Part model, mm, in its own coordinate system. A direction names the side the tool comes from. Coordinates: 2 decimals unless noted, no trailing zeros. Loops run counter-clockwise (first coordinate to the right, second up) from the corner with the lowest first, then second, coordinate; pieces in that order, holes last. Notation, with made-up numbers: (22, 22.25) -> (46, 22.25) arc R20 ccw to (46, 59.25) -> close; hole circle Ø4 at (-31, 39). An arc over 180 degrees is marked (long way). One line per question, with ' | ' between items. Start each with the question number.
1) Cut at B-B (z = -3.75). List the corners of the cut face in (x, y), plus the area to 3 significant figures.
2) Cut at D-D (y = 1.45). Count the separate pieces of the cut face and the enclosed holes in it, plus the area to 3 significant figures.
3) Cut at C-C (z = -49). List the corners of the cut face in (x, y).
4) Two-plate mould, pull along X, no slides. Class faces 1 (the face through (12, 3, -10)), 2 (the face through (70, 2, -35)), 3 (the face through (35, 2, -70)): released by +X, released by -X, zero draft, split by the parting line, or undercut.
5) 3-axis set-ups, long thin cutter, end or side, ignore diameter. For faces 4 (the face through (12, 3, -60)), 5 (the face through (35, 2, 0)): which of +Z, -Z, +X, -X, +Y, -Y reach the whole face in a straight line?
6) Probe L1, parallel to X at y = 3.45, z = -66.25; L2, parallel to X at y = 3.1, z = -46.5; L3, parallel to Z at x = 66.25, y = 1.5. List the from-to ranges inside material, lowest first. Write a range as from..to.
7) Cut at A-A (x = 66.25). List the corners of the cut face in (y, z), plus the area to 3 significant figures.
from build123d import *

# Parameters (mm, degrees)
SKETCH1_W                 = 70
SKETCH1_H                 = 70
BOSS_EXTRUDE1_DEPTH       = 5
SKETCH2_R                 = 1.25
CUT_EXTRUDE1_DEPTH        = 100.121138008
LPATTERN1_COUNT           = 2
LPATTERN1_PITCH           = 62.5
LPATTERN2_COUNT           = 2
LPATTERN2_PITCH           = 62.5
LPATTERN2_COPY_1_SKETCH_R = 1.25
LPATTERN2_COPY_1_DEPTH    = 100.121138008
SKETCH3_W                 = 5
SKETCH3_H                 = 50
CUT_EXTRUDE2_DEPTH        = 100.121138008
FILLET2_R                 = 1
FILLET3_R                 = 1
FILLET4_R                 = 1
FILLET5_R                 = 1
LPATTERN3_COUNT           = 5
LPATTERN3_PITCH           = 11.25
FILLET2_OF_LPATTERN3_R    = 1
FILLET3_OF_LPATTERN3_R    = 1
FILLET4_OF_LPATTERN3_R    = 1
FILLET5_OF_LPATTERN3_R    = 1
FILLET6_R                 = 1
FILLET7_R                 = 1
FILLET8_R                 = 1
FILLET9_R                 = 1
FILLET10_R                = 1


with BuildPart() as part:
    # Sketch1 → Boss-Extrude1 (new body)
    with BuildSketch(Plane(origin=(0, 0, 0), x_dir=(1, 0, 0), z_dir=(0, 1, 0))):
        with Locations((35, 35)):
            Rectangle(SKETCH1_W, SKETCH1_H)
    extrude(amount=BOSS_EXTRUDE1_DEPTH)

    # Sketch2 → Cut-Extrude1 (cut, through all)
    with BuildSketch(Plane(origin=(0, 5, 0), x_dir=(1, 0, 0), z_dir=(0, 1, 0))):
        with Locations(Location((3.75, 3.75, 0), (0, 0, 270))):
            Circle(SKETCH2_R)
    cut_extrude1 = extrude(amount=-CUT_EXTRUDE1_DEPTH, mode=Mode.SUBTRACT)

    # LPattern1: Cut-Extrude1 ×2
    with Locations(*[(i * LPATTERN1_PITCH, 0, 0) for i in range(1, LPATTERN1_COUNT)]):
        add(cut_extrude1, mode=Mode.SUBTRACT)

    # LPattern2: Cut-Extrude1 ×2
    with Locations(*[(0, 0, -i * LPATTERN2_PITCH) for i in range(1, LPATTERN2_COUNT)]):
        add(cut_extrude1, mode=Mode.SUBTRACT)

    # LPattern2 copy 1 sketch → LPattern2 copy 1 (cut, through all)
    with BuildSketch(Plane(origin=(62.5, 5, -62.5), x_dir=(1, 0, 0), z_dir=(0, 1, 0))):
        with Locations(Location((3.75, 3.75, 0), (0, 0, 270))):
            Circle(LPATTERN2_COPY_1_SKETCH_R)
    extrude(amount=-LPATTERN2_COPY_1_DEPTH, mode=Mode.SUBTRACT)

    # Sketch3 → Cut-Extrude2 (cut, through all)
    with BuildSketch(Plane(origin=(0, 5, 0), x_dir=(1, 0, 0), z_dir=(0, 1, 0))):
        with Locations((12.5, 35)):
            Rectangle(SKETCH3_W, SKETCH3_H)
    cut_extrude2 = extrude(amount=-CUT_EXTRUDE2_DEPTH, mode=Mode.SUBTRACT)

    # Fillet2
    fillet2_edges = [part.edges().sort_by_distance(p)[0] for p in [
        (10, 2.5, -60),
    ]]
    fillet(fillet2_edges, radius=FILLET2_R)

    # Fillet3
    fillet3_edges = [part.edges().sort_by_distance(p)[0] for p in [
        (15, 2.5, -60),
    ]]
    fillet(fillet3_edges, radius=FILLET3_R)

    # Fillet4
    fillet4_edges = [part.edges().sort_by_distance(p)[0] for p in [
        (10, 2.5, -10),
    ]]
    fillet(fillet4_edges, radius=FILLET4_R)

    # Fillet5
    fillet5_edges = [part.edges().sort_by_distance(p)[0] for p in [
        (15, 2.5, -10),
    ]]
    fillet(fillet5_edges, radius=FILLET5_R)

    # LPattern3: Cut-Extrude2 ×5
    with Locations(*[(i * LPATTERN3_PITCH, 0, 0) for i in range(1, LPATTERN3_COUNT)]):
        add(cut_extrude2, mode=Mode.SUBTRACT)

    # Fillet2 of LPattern3
    fillet2_of_lpattern3_edges = [part.edges().sort_by_distance(p)[0] for p in [
        (21.25, 2.5, -60),
        (32.5, 2.5, -60),
        (43.75, 2.5, -60),
        (55, 2.5, -60),
    ]]
    fillet(fillet2_of_lpattern3_edges, radius=FILLET2_OF_LPATTERN3_R)

    # Fillet3 of LPattern3
    fillet3_of_lpattern3_edges = [part.edges().sort_by_distance(p)[0] for p in [
        (26.25, 2.5, -60),
        (37.5, 2.5, -60),
        (48.75, 2.5, -60),
        (60, 2.5, -60),
    ]]
    fillet(fillet3_of_lpattern3_edges, radius=FILLET3_OF_LPATTERN3_R)

    # Fillet4 of LPattern3
    fillet4_of_lpattern3_edges = [part.edges().sort_by_distance(p)[0] for p in [
        (21.25, 2.5, -10),
        (32.5, 2.5, -10),
        (43.75, 2.5, -10),
        (55, 2.5, -10),
    ]]
    fillet(fillet4_of_lpattern3_edges, radius=FILLET4_OF_LPATTERN3_R)

    # Fillet5 of LPattern3
    fillet5_of_lpattern3_edges = [part.edges().sort_by_distance(p)[0] for p in [
        (26.25, 2.5, -10),
        (37.5, 2.5, -10),
        (48.75, 2.5, -10),
        (60, 2.5, -10),
    ]]
    fillet(fillet5_of_lpattern3_edges, radius=FILLET5_OF_LPATTERN3_R)

    # Fillet6
    fillet6_edges = [part.edges().sort_by_distance(p)[0] for p in [
        (70, 2.5, 0),
    ]]
    fillet(fillet6_edges, radius=FILLET6_R)

    # Fillet7
    fillet7_edges = [part.edges().sort_by_distance(p)[0] for p in [
        (0, 2.5, 0),
    ]]
    fillet(fillet7_edges, radius=FILLET7_R)

    # Fillet8
    fillet8_edges = [part.edges().sort_by_distance(p)[0] for p in [
        (0, 2.5, -70),
    ]]
    fillet(fillet8_edges, radius=FILLET8_R)

    # Fillet9
    fillet9_edges = [part.edges().sort_by_distance(p)[0] for p in [
        (70, 2.5, -70),
    ]]
    fillet(fillet9_edges, radius=FILLET9_R)

    # Fillet10
    fillet10_edges = [part.edges().sort_by_distance(p)[0] for p in [
        (70, 5, -35),
        (69.707106781, 5, -0.292893219),
        (35, 5, 0),
        (0.292893219, 5, -0.292893219),
        (0, 5, -35),
        (0.292893219, 5, -69.707106781),
        (35, 5, -70),
        (69.707106781, 5, -69.707106781),
    ]]
    fillet(fillet10_edges, radius=FILLET10_R)


solid = part.part
Reported:
1) outline: (0, 0) -> (2.5, 0) -> (2.5, 5) -> (1, 5) arc R1 ccw to (0, 4) -> close; (5, 0) -> (65, 0) -> (65, 5) -> (5, 5) -> close; (67.5, 0) -> (70, 0) -> (70, 4) arc R1 ccw to (69, 5) -> (67.5, 5) -> close | area: 325 mm²
2) separate pieces: 1 | enclosed holes: 9 | area: 3,630 mm²
3) outline: (0, 0) -> (10, 0) -> (10, 5) -> (1, 5) arc R1 ccw to (0, 4) -> close; (15, 0) -> (21.25, 0) -> (21.25, 5) -> (15, 5) -> close; (26.25, 0) -> (32.5, 0) -> (32.5, 5) -> (26.25, 5) -> close; (37.5, 0) -> (43.75, 0) -> (43.75, 5) -> (37.5, 5) -> close; (48.75, 0) -> (55, 0) -> (55, 5) -> (48.75, 5) -> close; (60, 0) -> (70, 0) -> (70, 4) arc R1 ccw to (69, 5) -> (60, 5) -> close
4) face 1: undercut | face 2: released by +X | face 3: zero draft
5) face 4: +Y, -Y | face 5: +Z, +X, -X, +Y, -Y
6) L1: x = 0..2.5, 5..65, 67.5..70 | L2: x = 0..10, 15..21.25, 26.25..32.5, 37.5..43.75, 48.75..55, 60..70 | L3: z = -70..-67.5, -65..-5, -2.5..0
7) outline: (0, -70) -> (4, -70) arc R1 ccw to (5, -69) -> (5, -67.5) -> (0, -67.5) -> close; (0, -65) -> (5, -65) -> (5, -5) -> (0, -5) -> close; (0, -2.5) -> (5, -2.5) -> (5, -1) arc R1 ccw to (4, 0) -> (0, 0) -> close | area: 325 mm²
